Check sheet for the modelled part. Datum: model origin and axes. Units: mm. A direction names the side the tool comes from. Give positions to 0.01 mm unless a question says otherwise; leave off trailing zeros. Order: outer loops, then holes, each group sorted by start corner. A loop starts at its lowest first (then second) coordinate and runs counter-clockwise, first axis right, second up. Notation, with made-up numbers: M -32,85.25 L -27,85.25 A23 ccw -27,96.25 Z; hole C 22,30.5 d1. An arc over 180 degrees is marked long. Answer in a Markdown table with one row per item. Add a question column.
from build123d import *

# Parameters (mm, degrees)
F0_W      = 431.8
F0_H      = 317.5
F1_DEPTH  = 1.27
F2_W      = 431.8
F2_H      = 1.27
F3_DEPTH  = 165.1
F4_R      = 1.27
F5_W      = 431.8
F5_H      = 1.27
F6_DEPTH  = 127
F7_R      = 1.27
F8_R      = 3.175
F9_DEPTH  = 25.4
F10_R     = 4.7625
F11_DEPTH = 317.501


with BuildPart() as f1:
    # F0 (on Front) → F1 (new body)
    with BuildSketch(Plane.XZ):
        with Locations((14.972474, 5.196487)):
            Rectangle(F0_W, F0_H)
    extrude(amount=F1_DEPTH)

    # F2 (on face) → F3 (join)
    with BuildSketch(Plane.XZ.offset(1.27)):
        with Locations((14.972474, 163.311487)):
            Rectangle(F2_W, F2_H)
    extrude(amount=F3_DEPTH)

    # F4
    f4_edges = [f1.edges().sort_by_distance(p)[0] for p in [
        (14.972474, -1.27, 162.676487),
        (14.972474, 0, 163.946487),
    ]]
    fillet(f4_edges, radius=F4_R)

    # F5 (on face) → F6 (join)
    with BuildSketch(Plane.XZ.offset(1.27)):
        with Locations((14.972474, -152.918513)):
            Rectangle(F5_W, F5_H)
    extrude(amount=F6_DEPTH)

    # F7
    f7_edges = [f1.edges().sort_by_distance(p)[0] for p in [
        (14.972474, -1.27, -152.283513),
        (14.972474, 0, -153.553513),
    ]]
    fillet(f7_edges, radius=F7_R)

    # F8 (on face) → F9 (cut)
    with BuildSketch(Plane.XZ.offset(1.27)):
        with Locations((-175.527526, 113.146487)):
            Circle(F8_R)
        with Locations((205.472474, 113.146487)):
            Circle(F8_R)
    extrude(amount=-F9_DEPTH, mode=Mode.SUBTRACT)

    # F10 (on face) → F11 (cut, through all)
    with BuildSketch(Plane.XY.offset(163.946487)):
        with Locations((-112.027526, -114.3)):
            Circle(F10_R)
        with Locations((141.972474, -114.3)):
            Circle(F10_R)
    extrude(amount=-F11_DEPTH, mode=Mode.SUBTRACT)


solid = f1.part
Q1. Thickness scan on probe 1 along Z at (x, y) = (16, -50.5); probe 2 along X at (y, z) = (-114, 163); probe 3 along Y at (x, z) = (-156.5, -135). Record the ranges inside material, lowest first.
Q2. Cross-section at C-C (x = -167.5). Record the boundary of the cut face in (y, z), and give its area (3 significant figures).
Q3. Cross-section at B-B (y = -114.3). Record the boundary of the cut face in (x, z), and give its area (3 significant figures).
Q4. Draft check along X on faces 1 (the cylindrical face through (-113.06, -118.95, 163.32)), 2 (the flat face through (12, -1.27, 7)). Enter one of: pulls with the +X half, pulls with the -X half, needs draft (parallel to the pull), parting line crosses it, or undercut.
Q5. Tool access check on faces 3 (the flat face through (12, -83, 162.676)), 4 (the cylindrical face through (146.372, -116.124, 163.32)). Record the directions out of +Z, -Z, +X, -X, +Y, -Y that give a thin tool (end or side, any length) a straight path to the whole face; none if there is none.
Q6. Go/stop test with flat-tipped pins: pin 1 (2 mm diameter, centred on x = -126, z = -112.5, fed in from -Y); pin 2 (0.6 mm diameter, centred on x = 39, z = -153, fed in from -Y); pin 3 (4 mm diameter, centred on x = -175.53, z = 113.15, fed in from -Y). Record where each tip stops, or that it passes through.
Q7. Cross-section at D-D (z = -95). Record the boundary of the cut face in (x, y), and give its area (3 significant figures).
Q8. Cross-section at A-A (y = -91.5). Record the boundary of the cut face in (x, z).
Values follow:
| question | item | result |
|---|---|---|
| 1 | probe 1 | -153.55 to -152.28, 162.68 to 163.95 |
| 1 | probe 2 | -200.93 to -116.78, -107.27 to 137.22, 146.73 to 230.87 |
| 1 | probe 3 | -1.27 to 0 |
| 2 | outline | M -166.37,162.68 L -2.54,162.68 A1.27 cw -1.27,161.41 L -1.27,-151.01 A1.27 cw -2.54,-152.28 L -128.27,-152.28 L -128.27,-153.55 L -1.27,-153.55 A1.27 ccw 0,-152.28 L 0,162.68 A1.27 ccw -1.27,163.95 L -166.37,163.95 Z |
| 2 | area | 774 mm² |
| 3 | outline | M -200.93,-153.55 L -116.79,-153.55 L -116.79,-152.28 L -200.93,-152.28 Z; M -200.93,162.68 L -116.79,162.68 L -116.79,163.95 L -200.93,163.95 Z; M -107.27,-153.55 L 137.21,-153.55 L 137.21,-152.28 L -107.27,-152.28 Z; M -107.27,162.68 L 137.21,162.68 L 137.21,163.95 L -107.27,163.95 Z; M 146.73,-153.55 L 230.87,-153.55 L 230.87,-152.28 L 146.73,-152.28 Z; M 146.73,162.68 L 230.87,162.68 L 230.87,163.95 L 146.73,163.95 Z |
| 3 | area | 1,050 mm² |
| 4 | face 1 | undercut |
| 4 | face 2 | needs draft |
| 5 | face 3 | +X, -X, -Y |
| 5 | face 4 | +Z, -Z |
| 6 | pin 1 | y = -1.27 |
| 6 | pin 2 | y = -128.27 |
| 6 | pin 3 | through |
| 7 | outline | M -200.93,-1.27 L 230.87,-1.27 L 230.87,0 L -200.93,0 Z |
| 7 | area | 548 mm² |
| 8 | outline | M -200.93,-153.55 L 230.87,-153.55 L 230.87,-152.28 L -200.93,-152.28 Z; M -200.93,162.68 L 230.87,162.68 L 230.87,163.95 L -200.93,163.95 Z |
